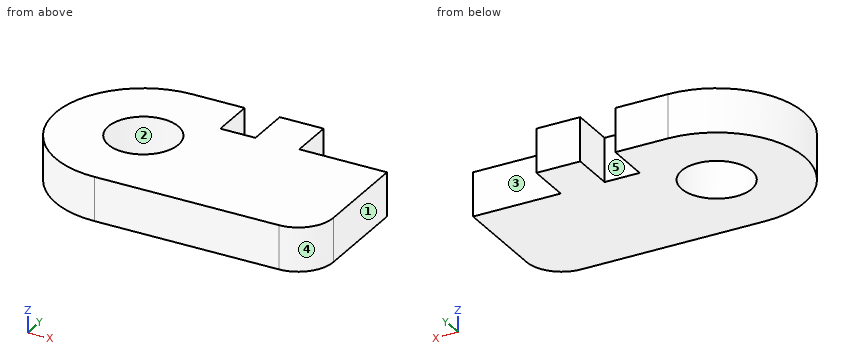
from build123d import *

# Parameters (mm, degrees)
SKETCH1_R           = 4
BOSS_EXTRUDE4_DEPTH = 5


with BuildPart() as part:
    # Sketch1 → Boss-Extrude4 (new body)
    with BuildSketch(Plane.XY):
        with BuildLine():
            Line((22.5, 5), (22.5, -6))
            ThreePointArc((22.5, -6), (21.328427125, -8.828427125), (18.5, -10))
            Line((18.5, -10), (-2.5, -10))
            ThreePointArc((-2.5, -10), (-12.5, 0), (-2.5, 10))
            Line((-2.5, 10), (3.5, 10))
            Line((3.5, 10), (3.5, 5))
            Line((3.5, 5), (7.5, 5))
            Line((7.5, 5), (7.5, 10))
            Line((7.5, 10), (12.5, 10))
            Line((12.5, 10), (12.5, 5))
            Line((12.5, 5), (22.5, 5))
        make_face()
        with Locations((-2.5, 0)):
            Circle(SKETCH1_R, mode=Mode.SUBTRACT)
    extrude(amount=BOSS_EXTRUDE4_DEPTH)


solid = part.part
Model file for the job. Use its own axes, mm. Face numbers are marked on the shaded views. A direction names the side the tool comes from. Give positions to 0.01 mm unless a question says otherwise; leave off trailing zeros. Order: outer loops, then holes, each group sorted by start corner. A loop starts at its lowest first (then second) coordinate and runs counter-clockwise, first axis right, second up. Notation, with made-up numbers: M 20.25,39 L 45.25,39 A15 cw 45.25,62 Z; hole C 20.25,-26 d5. An arc over 180 degrees is marked long. Put each result on its own line as item: value. Start each with the question number.
(1) Band-saw the part on C-C on y = 7. Give the cut face in (x, z).
(2) Band-saw the part on B-B on z = 3.3. Give the cut face in (x, y).
(3) Pull direction X, two halves, no side cores. Call the marked faces 1, 2 and 3: released by +X, released by -X, zero draft, split by the parting line, or undercut.
(4) Band-saw the part on D-D on x = 5. Give the cut face in (y, z).
(5) Pin check, flat tips, straight feed: pin 1 Ø2.5 at (y, z) = (6.5, 2) entering from +X; pin 2 Ø6.5 at (x, y) = (-2.5, 0) entering from -Z; pin 3 Ø1.2 at (x, z) = (4.5, 3) entering from +Y. Stop position of each tip, or through.
(6) Band-saw the part on A-A on y = 0. Give the cut face in (x, z), then the cut area to 3 significant figures.
(7) Drill centre lines: L1, parallel to Y at x = -2.5, z = 2.3; L2, parallel to X at y = -3, z = 4; L3, parallel to Y at x = 16, z = 4.4. Where is each one in solid material? Low to high. Write a range as [from, to].
(8) Tool access for the marked faces 4 and 5: list every direction of +Z, -Z, +X, -X, +Y, -Y with a clear straight run to the whole face (end or side of a thin tool).
Results below:
1. outline: M -9.64,0 L 3.5,0 L 3.5,5 L -9.64,5 Z; M 7.5,0 L 12.5,0 L 12.5,5 L 7.5,5 Z
2. outline: M -2.5,-10 L 18.5,-10 A4 ccw 22.5,-6 L 22.5,5 L 12.5,5 L 12.5,10 L 7.5,10 L 7.5,5 L 3.5,5 L 3.5,10 L -2.5,10 A10 ccw Z; hole C -2.5,0 d8
3. face 1: released by +X
3. face 2: undercut
3. face 3: zero draft
4. outline: M -10,0 L 5,0 L 5,5 L -10,5 Z
5. pin 1: stops at x = 12.5
5. pin 2: passes through
5. pin 3: stops at y = 5
6. outline: M -12.5,0 L -6.5,0 L -6.5,5 L -12.5,5 Z; M 1.5,0 L 22.5,0 L 22.5,5 L 1.5,5 Z
6. area: 135 mm2
7. L1: y = [-10, -4], [4, 10]
7. L2: x = [-12.04, -5.15], [0.15, 22.5]
7. L3: y = [-10, 5]
8. face 4: +Z, -Z, +X, -Y
8. face 5: +Z, -Z, +Y
